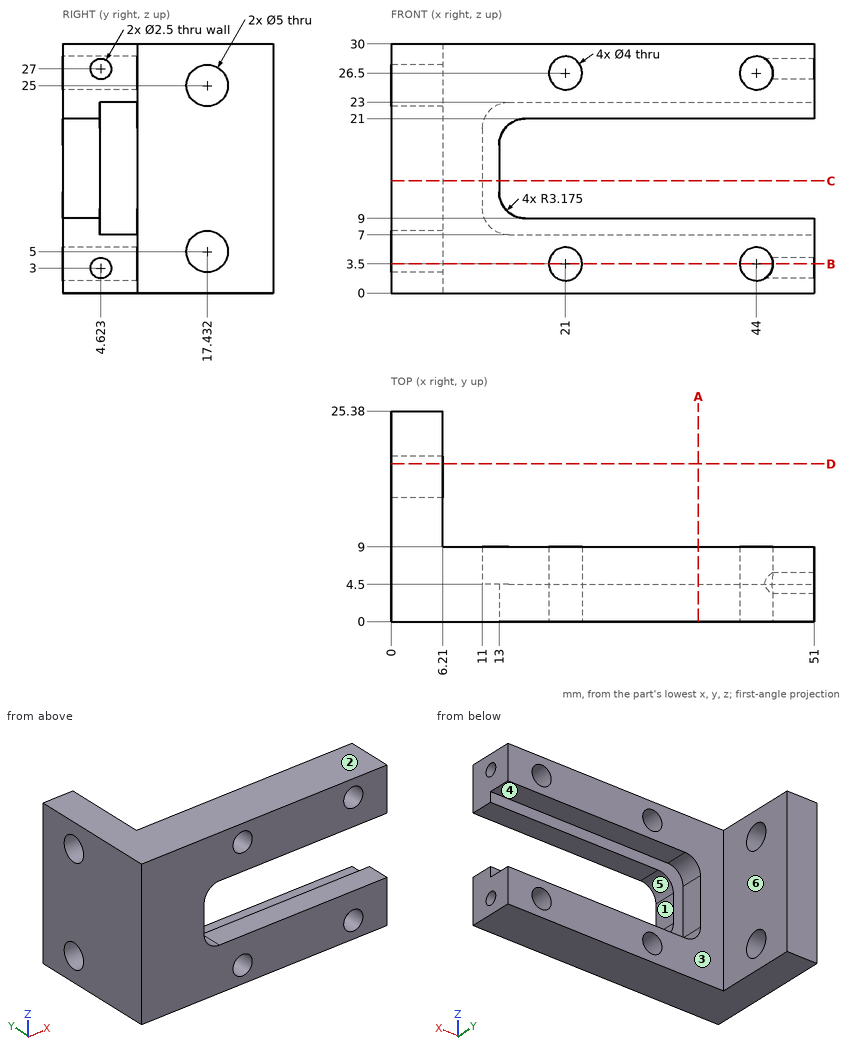
Answer from the drawing. Dimensions are ordinates in mm from the lowest x, y and z of the part. A direction names the side the tool comes from. Round coordinates to 2 decimals unless told otherwise and drop trailing zeros. Write each loop counter-clockwise with the first axis right and the second up, starting at its lowest first coordinate (ties: lowest second). Pieces come first, ordered by that corner, then holes. Notation, with made-up numbers: M 44.25,58.25 L 94.25,58.25 A20 cw 94.25,79.25 Z; hole C -32.75,80 d11. An arc over 180 degrees is marked long. Write each question's results on one line, items separated by ' | '. Start each with the question number.
Item 1: Straight lines are drawn through the part: L1, parallel to Z at x = 44, y = 6; L2, parallel to Z at x = 44, y = 4; L3, parallel to Z at x = 26, y = 3.25. For each, find the intervals that lie inside material, in ascending order. Write a range as [from, to].
Item 2: A cutting plane is placed at D-D on y = 19. Write down the section's boundary in (x, z), and give its area (3 significant figures).
Item 3: A cutting plane is placed at B-B on z = 3.5. Write down the section's boundary in (x, y).
Item 4: For the marked faces 4, 5 and 6, determine the directions among +Z, -Z, +X, -X, +Y, -Y from which every point of the face is accessible in a straight line to the end or side of a thin tool.
Item 5: Flat-ended cylindrical pins translate along their axes: pin 1 Ø5 at (y, z) = (19, 14.5) entering from +X; pin 2 Ø3.5 at (y, z) = (6.5, 16.5) entering from +X; pin 3 Ø4 at (y, z) = (17.43, 25) entering from -X; pin 4 Ø4.5 at (x, z) = (21, 26.5) entering from +Y. Find the tip coordinate at first contact, or state that the pin passes through.
Item 6: For a pull along Z with two mould halves and no side action, classify the marked faces 1, 2 and 3 as pulls with the +Z half, pulls with the -Z half, needs draft (parallel to the pull), parting line crosses it, or undercut.
Item 7: A cutting plane is placed at C-C on z = 13.5. Write down the section's boundary in (x, y), and give its area (3 significant figures).
Item 8: A cutting plane is placed at A-A on x = 37. Write down the section's boundary in (y, z).
Check sheet entries:
1) L1: [0, 1.5], [5.5, 7], [23, 24.5], [28.5, 30] | L2: [0, 1.5], [5.5, 9], [21, 24.5], [28.5, 30] | L3: [0, 9], [21, 30]
2) outline: M 0,0 L 6.21,0 L 6.21,3.05 L 0,3.05 Z; M 0,6.95 L 6.21,6.95 L 6.21,23.05 L 0,23.05 Z; M 0,26.95 L 6.21,26.95 L 6.21,30 L 0,30 Z | area: 138 mm²
3) outline: M 0,0 L 19,0 L 19,9 L 6.21,9 L 6.21,15.43 L 0,15.43 Z; M 0,19.43 L 6.21,19.43 L 6.21,25.38 L 0,25.38 Z; M 23,0 L 42,0 L 42,9 L 23,9 Z; M 46,0 L 51,0 L 51,3.48 L 46,3.48 Z; M 46,5.77 L 51,5.77 L 51,9 L 46,9 Z
4) face 4: +X, +Y | face 5: +X, +Y, -Y | face 6: +Z, -Z, +X, +Y
5) pin 1: x = 6.21 | pin 2: x = 11 | pin 3: through | pin 4: y = 9
6) face 1: undercut | face 2: pulls with the +Z half | face 3: needs draft
7) outline: M 0,0 L 13,0 L 13,4.5 L 11,4.5 L 11,9 L 6.21,9 L 6.21,25.38 L 0,25.38 Z | area: 210 mm²
8) outline: M 0,0 L 9,0 L 9,7 L 4.5,7 L 4.5,9 L 0,9 Z; M 0,21 L 4.5,21 L 4.5,23 L 9,23 L 9,30 L 0,30 Z
